from build123d import *

# Parameters (mm, degrees)
F1_DEPTH  = 131.8250094
F2_W      = 9.525
F2_H      = 119.1250094
F3_DEPTH  = 108.98632
F4_R      = 3.69316
F5_R      = 1.98374
F6_R      = 1.8288
F7_DEPTH  = 257
F8_R      = 2.5
F9_DEPTH  = 1.70942
F10_R     = 1.35255
F11_DEPTH = 1.70942


# Not quite as in the source:
# - an extrude ends at something that could not be found from the text; its depth is read off the source's solid


with BuildPart() as f1:
    # F0 (on Top) → F1 (new body)
    with BuildSketch(Plane.XY):
        Polygon((0, 16.27124), (0, 0), (-105.56748, 0), (-105.56748, 16.27124), (-107.2769, 16.27124), (-107.2769, -1.70942), (1.70942, -1.70942), (1.70942, 16.27124), align=None)
    extrude(amount=F1_DEPTH)

    # F2 (on face) → F3 (cut, through all)
    with BuildSketch(Plane.YZ.offset(1.70942)):
        with Locations((8.33374, 65.9125047)):
            Rectangle(F2_W, F2_H)
    extrude(amount=-F3_DEPTH, mode=Mode.SUBTRACT)

    # F4
    f4_edges = [f1.edges().sort_by_distance(p)[0] for p in [
        (1.70942, -1.70942, 65.912505),
        (-107.2769, -1.70942, 65.912505),
    ]]
    fillet(f4_edges, radius=F4_R)

    # F5
    f5_edges = [f1.edges().sort_by_distance(p)[0] for p in [
        (0, 0, 65.912505),
        (-105.56748, 0, 65.912505),
    ]]
    fillet(f5_edges, radius=F5_R)

    # F6 (on face) → F7 (cut, through all)
    with BuildSketch(Plane.XZ.offset(1.70942)):
        with Locations((-52.78374, 120.65)):
            Circle(F6_R)
        with Locations((-5.15874, 120.65)):
            Circle(F6_R)
        with Locations((-100.40874, 120.65)):
            Circle(F6_R)
        with Locations((-45.63999, 3.175)):
            Circle(F6_R)
        with Locations((-59.92749, 3.175)):
            Circle(F6_R)
    extrude(amount=-F7_DEPTH, mode=Mode.SUBTRACT)

    # F8 (on face) → F9 (cut, through all)
    with BuildSketch(Plane.XZ.offset(1.70942)):
        with Locations((-8.452485, 127.8250094)):
            Circle(F8_R)
        with Locations((-8.452485, 4)):
            Circle(F8_R)
        with Locations((-97.114995, 4)):
            Circle(F8_R)
        with Locations((-97.114995, 127.8250094)):
            Circle(F8_R)
    extrude(amount=-F9_DEPTH, mode=Mode.SUBTRACT)

    # F10 (on face) → F11 (cut, through all)
    with BuildSketch(Plane.XZ.offset(1.70942)):
        with Locations((-43.25874, 57.9750047)):
            Circle(F10_R)
        with Locations((-43.25874, 73.8500047)):
            Circle(F10_R)
        with Locations((-62.30874, 57.9750047)):
            Circle(F10_R)
        with Locations((-62.30874, 73.8500047)):
            Circle(F10_R)
    extrude(amount=-F11_DEPTH, mode=Mode.SUBTRACT)


solid = f1.part
The model under review builds one solid part; all positions refer to its coordinate system, in mm. Round coordinates to 2 decimals unless told otherwise and drop trailing zeros. Write each loop counter-clockwise with the first axis right and the second up, starting at its lowest first coordinate (ties: lowest second). Pieces come first, ordered by that corner, then holes. Notation, with made-up numbers: M 7.25,53 L 21.25,53 A9 ccw 21.25,68 Z; hole C 28.25,45.5 d3. An arc over 180 degrees is marked long. Use a Markdown table: item, result. Add a question column.
Q1. Insertion check: pin 1 (1.5 mm diameter, centred on x = -22, z = 84.5, fed in from +Y); pin 2 (1.9 mm diameter, centred on x = 1, z = 85, fed in from -Y); pin 3 (1.4 mm diameter, centred on x = -107, z = 52.5, fed in from -Y); pin 4 (2 mm diameter, centred on x = -43.26, z = 57.98, fed in from -Y). Each pin has a flat end and moves straight along its axis. Give the tip position at first contact, or say it passes through.
Q2. We need section B-B, the plane y = 5.5. State the section outline as (x, z) points (3 decimals), plus the area to 3 significant figures.
Q3. We need section C-C, the plane z = 94.5. State the section outline as (x, y) points, plus the area to 3 significant figures.
Q4. To check wall thickness, follow line 1 (X direction, y = 2.75, z = 87); line 2 (X direction, y = -1.15, z = 120.65); line 3 (X direction, y = -0.7, z = 120.65). State the ranges of each line that lie inside material, in increasing order.
Q5. We need section D-D, the plane x = -26.5. State the section outline as (y, z) points (3 decimals).
Q6. We need section A-A, the plane z = 120.65. Count the separate pieces of the cut face and the enclosed holes in it, plus the area to 3 significant figures.
Q7. The part is to be moulded in two halves that separate along X. For faces 1 (the face through (-53, -1, 131.825)), 2 (the face through (0.656, -0.599, 66.835)), 3 (the face through (0, 14, 66)), say which applies: pulls with the +X half, pulls with the -X half, needs draft (parallel to the pull), parting line crosses it, or undercut.
Findings below:
| question | item | result |
|---|---|---|
| 1 | pin 1 | stops at y = 0 |
| 1 | pin 2 | stops at y = -1.1 |
| 1 | pin 3 | stops at y = -0.52 |
| 1 | pin 4 | passes through |
| 2 | outline | M -107.277,0 L -105.567,0 L -105.567,6.35 L -107.277,6.35 Z; M -107.277,125.475 L -105.567,125.475 L -105.567,131.825 L -107.277,131.825 Z; M 0,0 L 1.709,0 L 1.709,6.35 L 0,6.35 Z; M 0,125.475 L 1.709,125.475 L 1.709,131.825 L 0,131.825 Z |
| 2 | area | 43.4 mm² |
| 3 | outline | M -107.28,1.98 A3.69 ccw -103.58,-1.71 L -1.98,-1.71 A3.69 ccw 1.71,1.98 L 1.71,3.57 L 0,3.57 L 0,1.98 A1.98 cw -1.98,0 L -103.58,0 A1.98 cw -105.57,1.98 L -105.57,3.57 L -107.28,3.57 Z; M -107.28,13.1 L -105.57,13.1 L -105.57,16.27 L -107.28,16.27 Z; M 0,13.1 L 1.71,13.1 L 1.71,16.27 L 0,16.27 Z |
| 3 | area | 205 mm² |
| 4 | line 1 | x = -107.28 to -105.57, 0 to 1.71 |
| 4 | line 2 | x = -105.54 to -102.24, -98.58 to -54.61, -50.95 to -6.99, -3.33 to -0.03 |
| 4 | line 3 | x = -106.12 to -102.24, -98.58 to -54.61, -50.95 to -6.99, -3.33 to 0.55 |
| 5 | outline | M -1.709,0 L 0,0 L 0,131.825 L -1.709,131.825 Z |
| 6 | separate pieces | 6 |
| 6 | enclosed holes | 0 |
| 6 | area | 186 mm² |
| 7 | face 1 | needs draft |
| 7 | face 2 | pulls with the +X half |
| 7 | face 3 | undercut |
